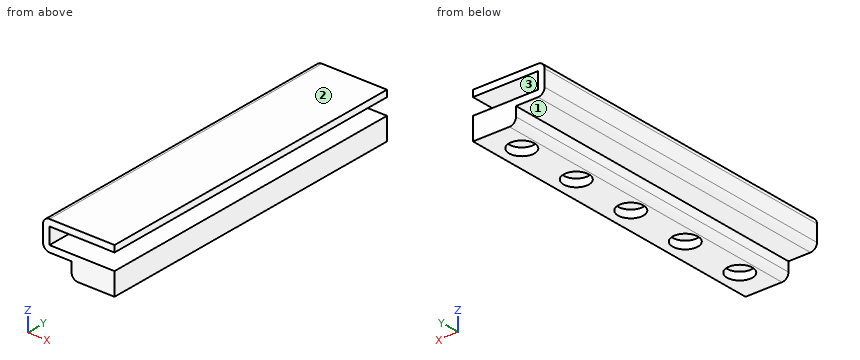
Autodesk Inventor part; units mm, degrees
ref_plane "YZ Plane" through (0, 0, 0) normal (1, 0, 0) x (0, 1, 0)
ref_plane "XZ Plane" through (0, 0, 0) normal (0, 1, 0) x (-1, 0, 0)
ref_plane "XY Plane" through (0, 0, 0) normal (0, 0, 1) x (1, 0, 0)
sketch "Sketch1" plane through (0, 0, 0) normal (0, 1, 0) x (-1, 0, 0)
  line L0 (0, 0) -> (25.4, 0)
  line L1 (25.4, 0) -> (25.4, 2.54)
  line L2 (25.4, 2.54) -> (0, 2.54)
  line L3 (0, 2.54) -> (0, 0)
  line L4 (25.4, 2.54) -> (27.94, 2.54)
  line L5 (27.94, 2.54) -> (27.94, -8.89)
  line L6 (27.94, -8.89) -> (25.4, -8.89)
  line L7 (25.4, -8.89) -> (25.4, 2.54)
  line L8 (-1.2994, 2.54) -> (27.94, 2.54)
  line L9 (25.4, -8.89) -> (0, -8.89)
  line L10 (0, -8.89) -> (0, -6.35)
  line L11 (0, -6.35) -> (25.4, -6.35)
  line L12 (25.4, -6.35) -> (25.4, -8.89)
  line L13 (8.3183, -8.89) -> (0, -8.89)
  line L14 (0, -8.89) -> (0, -12.3973)
  line L15 (0, -12.3973) -> (8.3183, -12.3973)
  line L16 (8.3183, -12.3973) -> (8.3183, -8.89)
  line L17 (0, -12.3973) -> (0, -6.35)
  line L18 (8.3183, -12.3973) -> (16.7954, -12.3973)
  line L19 (16.7954, -12.3973) -> (16.7954, -8.89)
  line L20 (16.7954, -8.89) -> (8.3183, -8.89)
  line L21 (8.3183, -8.89) -> (8.3183, -12.3973)
  line L22 (0, -12.3973) -> (16.7954, -12.3973)
  line L23 (16.7954, -12.3973) -> (16.7954, -15.1027)
  line L24 (16.7954, -15.1027) -> (0, -15.1027)
  line L25 (0, -15.1027) -> (0, -12.3973)
  point P0 (26.67, 2.54)
  point P1 (26.67, -8.89)
  point P2 (0, -8.89)
  point P3 (0, -8.89)
  dimension "d0" = 25.4
  dimension "d1" = 2.54
  dimension "d2" = 2.54
  dimension "d3" = 11.43
  dimension "d4" = 2.54
extrude "Extrusion1" add sketch "Sketch1" along normal blind 127
sketch "Sketch4" plane through (0, 0, -15.1027) normal (0, 0, -1) x (-1, 0, 0)
  circle A0 centre (8.4134, 114.3) radius 4.95
  line L0 (16.7954, 0) -> (16.7954, 127)
  circle A1 centre (8.4134, 88.9) radius 4.95
  circle A2 centre (8.4134, 63.5) radius 4.95
  circle A3 centre (8.4134, 38.1) radius 4.95
  circle A4 centre (8.4134, 12.7) radius 4.95
  line L1 (0, 127) -> (16.7954, 127)
  point P0 (0, 0)
  dimension "d15" = 9.9
  dimension "d16" = 8.382
  dimension "d19" = 25.4
  dimension "d24" = 12.7
extrude "Extrusion3" cut sketch "Sketch4" against normal blind 3
fillet "Fillet3" radius 2.54 3 edges at (-27.94, 63.5, -8.89) (-27.94, 63.5, 2.54) (-16.7954, 63.5, -15.1027)
properties part number "magnet"
Build history of the part. All positions in model axes, mm. Face numbers are marked on the shaded views. A direction names the side the tool comes from. Round coordinates to 2 decimals unless told otherwise and drop trailing zeros. Loops run counter-clockwise (first coordinate to the right, second up) from the corner with the lowest first, then second, coordinate; pieces in that order, holes last. Notation, with made-up numbers: (38, -38.75) -> (97, -38.75) arc R31 cw to (97, -1.75) -> close; hole circle Ø3 at (21.5, 74). An arc over 180 degrees is marked (long way). Use CSV: the item, a comma, the result in double quotes. Start each with the question number.
Q1. Drill centre lines: L1, parallel to Z at x = -7.5, y = 121; L2, parallel to Z at x = -21, y = 90; L3, parallel to X at y = 106.5, z = -0.75. Where is each one in solid material? Low to high.
Q2. Flat gauge pins, fed straight in: pin 1 Ø3 at (x, y) = (-8, 13.5) entering from -Z; pin 2 Ø2.5 at (x, y) = (-20.5, 34.5) entering from -Z; pin 3 Ø5 at (y, z) = (84, -3.5) entering from +X. Where does each tip first touch, or does it go through?
Q3. Saw through at D-D on z = -2. Give the cut face in (x, y).
Q4. Saw through at B-B on x = -7.75. Give the cut face in (y, z), and give its area (3 significant figures).
Q5. Which spindle directions (+Z, -Z, +X, -X, +Y, -Y) get a long thin tool onto all of the face, cutting with end or side? Do the marked faces 1, 2 and 3. Say none if no direction does.
Q6. Saw through at A-A on y = 76. Give the cut face in (x, z).
Q7. Saw through at C-C on z = -14. Give the cut face in (x, y).
Solutions:
1,L1,"z = -15.1 to -6.35, 0 to 2.54"
1,L2,"z = -8.89 to -6.35, 0 to 2.54"
1,L3,"x = -27.94 to -25.4"
2,pin 1,"stops at z = -12.1"
2,pin 2,"stops at z = -8.89"
2,pin 3,"stops at x = -25.4"
3,outline,"(-27.94, 0) -> (-25.4, 0) -> (-25.4, 127) -> (-27.94, 127) -> close"
4,outline,"(0, -15.1) -> (7.79, -15.1) -> (7.79, -12.1) -> (17.61, -12.1) -> (17.61, -15.1) -> (33.19, -15.1) -> (33.19, -12.1) -> (43.01, -12.1) -> (43.01, -15.1) -> (58.59, -15.1) -> (58.59, -12.1) -> (68.41, -12.1) -> (68.41, -15.1) -> (83.99, -15.1) -> (83.99, -12.1) -> (93.81, -12.1) -> (93.81, -15.1) -> (109.39, -15.1) -> (109.39, -12.1) -> (119.21, -12.1) -> (119.21, -15.1) -> (127, -15.1) -> (127, -6.35) -> (0, -6.35) -> close; (0, 0) -> (127, 0) -> (127, 2.54) -> (0, 2.54) -> close"
4,area,"1,290 mm^2"
5,face 1,"-Z, -X, +Y, -Y"
5,face 2,"+Z, +X, -X, +Y, -Y"
5,face 3,"+X, +Y, -Y"
6,outline,"(-27.94, -6.35) arc R2.54 ccw to (-25.4, -8.89) -> (-16.8, -8.89) -> (-16.8, -12.56) arc R2.54 ccw to (-14.26, -15.1) -> (0, -15.1) -> (0, -6.35) -> (-25.4, -6.35) -> (-25.4, 0) -> (0, 0) -> (0, 2.54) -> (-25.4, 2.54) arc R2.54 ccw to (-27.94, 0) -> close"
7,outline,"(-16.35, 0) -> (0, 0) -> (0, 127) -> (-16.35, 127) -> close; hole circle Ø9.9 at (-8.41, 12.7); hole circle Ø9.9 at (-8.41, 38.1); hole circle Ø9.9 at (-8.41, 63.5); hole circle Ø9.9 at (-8.41, 88.9); hole circle Ø9.9 at (-8.41, 114.3)"
